Here's how the part is built. I have some questions about the finished solid (model axes, mm). Give positions to 0.01 mm unless a question says otherwise; leave off trailing zeros. Write each loop counter-clockwise with the first axis right and the second up, starting at its lowest first coordinate (ties: lowest second). Pieces come first, ordered by that corner, then holes. Notation, with made-up numbers: (4, 74) -> (33, 74) arc R28 ccw to (33, 103) -> close; hole circle Ø2 at (8.5, -11). An arc over 180 degrees is marked (long way). Use one line per item in the form item = value.
```python
from build123d import *

# Parameters (mm, degrees)
SKETCH1_R               = 1.778
BOSS_EXTRUDE1_DEPTH     = 6.35
CUT_EXTRUDE1_DEPTH      = 103.859220114
CUT_EXTRUDE1_DEPTH_BACK = 103.859220114
SKETCH3_W               = 243.845776737
SKETCH3_H               = 94.534413445
CUT_EXTRUDE2_DEPTH      = 3.175


with BuildPart() as part:
    # Sketch1 → Boss-Extrude1 (new body)
    with BuildSketch(Plane(origin=(0, 6.35, 0), x_dir=(1, 0, 0), z_dir=(0, 1, 0))):
        with BuildLine():
            Line((97.79, 4.7625), (-97.79, 4.7625))
            ThreePointArc((-97.79, 4.7625), (-102.5525, 0), (-97.79, -4.7625))
            Line((-97.79, -4.7625), (97.79, -4.7625))
            ThreePointArc((97.79, -4.7625), (102.5525, 0), (97.79, 4.7625))
        make_face()
        with Locations(Location((97.79, 0, 0), (0, 0, 90))):
            Circle(SKETCH1_R, mode=Mode.SUBTRACT)
        with Locations(Location((88.011, 0, 0), (0, 0, 90))):
            Circle(SKETCH1_R, mode=Mode.SUBTRACT)
        with Locations(Location((78.232, 0, 0), (0, 0, 90))):
            Circle(SKETCH1_R, mode=Mode.SUBTRACT)
        with Locations(Location((68.453, 0, 0), (0, 0, 90))):
            Circle(SKETCH1_R, mode=Mode.SUBTRACT)
        with Locations(Location((58.674, 0, 0), (0, 0, 90))):
            Circle(SKETCH1_R, mode=Mode.SUBTRACT)
        with Locations(Location((48.895, 0, 0), (0, 0, 90))):
            Circle(SKETCH1_R, mode=Mode.SUBTRACT)
        with Locations(Location((39.116, 0, 0), (0, 0, 90))):
            Circle(SKETCH1_R, mode=Mode.SUBTRACT)
        with Locations(Location((29.337, 0, 0), (0, 0, 90))):
            Circle(SKETCH1_R, mode=Mode.SUBTRACT)
        with Locations(Location((19.558, 0, 0), (0, 0, 90))):
            Circle(SKETCH1_R, mode=Mode.SUBTRACT)
        with Locations(Location((9.779, 0, 0), (0, 0, 90))):
            Circle(SKETCH1_R, mode=Mode.SUBTRACT)
        with Locations(Location((0, 0, 0), (0, 0, 90))):
            Circle(SKETCH1_R, mode=Mode.SUBTRACT)
        with Locations(Location((-9.779, 0, 0), (0, 0, 90))):
            Circle(SKETCH1_R, mode=Mode.SUBTRACT)
        with Locations(Location((-19.558, 0, 0), (0, 0, 90))):
            Circle(SKETCH1_R, mode=Mode.SUBTRACT)
        with Locations(Location((-29.337, 0, 0), (0, 0, 90))):
            Circle(SKETCH1_R, mode=Mode.SUBTRACT)
        with Locations(Location((-39.116, 0, 0), (0, 0, 90))):
            Circle(SKETCH1_R, mode=Mode.SUBTRACT)
        with Locations(Location((-48.895, 0, 0), (0, 0, 90))):
            Circle(SKETCH1_R, mode=Mode.SUBTRACT)
        with Locations(Location((-58.674, 0, 0), (0, 0, 90))):
            Circle(SKETCH1_R, mode=Mode.SUBTRACT)
        with Locations(Location((-68.453, 0, 0), (0, 0, 90))):
            Circle(SKETCH1_R, mode=Mode.SUBTRACT)
        with Locations(Location((-78.232, 0, 0), (0, 0, 90))):
            Circle(SKETCH1_R, mode=Mode.SUBTRACT)
        with Locations(Location((-88.011, 0, 0), (0, 0, 90))):
            Circle(SKETCH1_R, mode=Mode.SUBTRACT)
        with Locations(Location((-97.79, 0, 0), (0, 0, 90))):
            Circle(SKETCH1_R, mode=Mode.SUBTRACT)
    extrude(amount=-BOSS_EXTRUDE1_DEPTH)

    # Sketch2 → Cut-Extrude1 (cut, two sides: drawn at the far end of the back side and taken through both)
    with BuildSketch(Plane(origin=(0, 6.35, 0), x_dir=(1, 0, 0), z_dir=(0, 1, 0)).offset(-CUT_EXTRUDE1_DEPTH_BACK)):
        with BuildLine():
            Line((-68.453, -4.7625), (-109.387336875, -4.7625))
            Line((-109.387336875, -4.7625), (-109.387336875, 4.7625))
            Line((-109.387336875, 4.7625), (-68.453, 4.7625))
            ThreePointArc((-68.453, 4.7625), (-73.2155, 0), (-68.453, -4.7625))
        make_face()
    extrude(amount=CUT_EXTRUDE1_DEPTH + CUT_EXTRUDE1_DEPTH_BACK, mode=Mode.SUBTRACT)

    # Sketch3 → Cut-Extrude2 (cut)
    with BuildSketch(Plane(origin=(0, 6.35, 0), x_dir=(1, 0, 0), z_dir=(0, 1, 0))):
        with Locations((-6.250363069, -2.208747977)):
            Rectangle(SKETCH3_W, SKETCH3_H)
    extrude(amount=-CUT_EXTRUDE2_DEPTH, mode=Mode.SUBTRACT)


solid = part.part
```
Q1. If we mould it in two halves opening along Z, with no side actions, what happens to faces 1 (the face through (16, 2, -4.762)), 2 (the face through (-8, 2, 0)), 3 (the face through (-73.214, 1.565, -0.105))? For each: +Z half, -Z half, draft (parallel to the pull), parting line (faces both ways), or undercut.
Result set:
face_1 = -Z half
face_2 = undercut
face_3 = parting line
Q2. Will this pin go through, and if not, where does the flat tip stop? pin 1 Ø1 at (y, z) = (1, 1) entering from -X.
Result set:
pin_1 = -73.19
Q3. I want a section at A-A, the plane x = 0. Write out the boundary of the cut face in (y, z) (1 decimal).
Result set:
outline = (0, -4.8) -> (3.2, -4.8) -> (3.2, -1.8) -> (0, -1.8) -> close; (0, 1.8) -> (3.2, 1.8) -> (3.2, 4.8) -> (0, 4.8) -> close
Q4. If I drill on line 1 along Z through (x, y) = (29.5, 1.55); line 2 along Z through (x, y) = (89, 2.2); line 3 along X through (y, z) = (1.55, 3), over which ranges is the centre line in solid material (lowest first)? Write a range as from..to.
Result set:
line_1 = -4.76..-1.77, 1.77..4.76
line_2 = -4.76..-1.48, 1.48..4.76
line_3 = -72.15..101.49
Q5. I want a section at B-B, the plane y = 1.75. Count the separate pieces of the cut face and the enclosed holes in it, and give its area (3 significant figures).
Result set:
separate_pieces = 1
enclosed_holes = 18
area = 1,480 mm2
